```python
from build123d import *

# Parameters (mm, degrees)
ESQUISSE1_R             = 4
BASE_EXTRUSION_DEPTH    = 25
ESQUISSE2_R             = 6.5
BOSS_EXTRU_1_DEPTH      = 8
ENL_V_MAT_EXTRU_1_DEPTH = 3.5
CONG_2_R                = 0.5
CHANFREIN1_SIZE         = 0.5


with BuildPart() as part:
    # Esquisse1 → Base-Extrusion (new body)
    with BuildSketch(Plane.XY):
        Circle(ESQUISSE1_R)
    extrude(amount=BASE_EXTRUSION_DEPTH)

    # Esquisse2 → Boss.-Extru.1 (add)
    with BuildSketch(Plane.XY.offset(25)):
        Circle(ESQUISSE2_R)
    extrude(amount=BOSS_EXTRU_1_DEPTH)

    # Esquisse3 → Enlèv. mat.-Extru.1 (cut)
    with BuildSketch(Plane.XY.offset(33)):
        Polygon((-1.732050808, 3), (1.732050808, 3), (3.464101615, 0), (1.732050808, -3), (-1.732050808, -3), (-3.464101615, 0), align=None)
    extrude(amount=-ENL_V_MAT_EXTRU_1_DEPTH, mode=Mode.SUBTRACT)

    # Congé2
    cong_2_edges = [part.edges().sort_by_distance(p)[0] for p in [
        (-6.5, 0, 33),
    ]]
    fillet(cong_2_edges, radius=CONG_2_R)

    # Chanfrein1
    chanfrein1_edges = [part.edges().sort_by_distance(p)[0] for p in [
        (-4, 0, 0),
    ]]
    chamfer(chanfrein1_edges, length=CHANFREIN1_SIZE)


solid = part.part
```
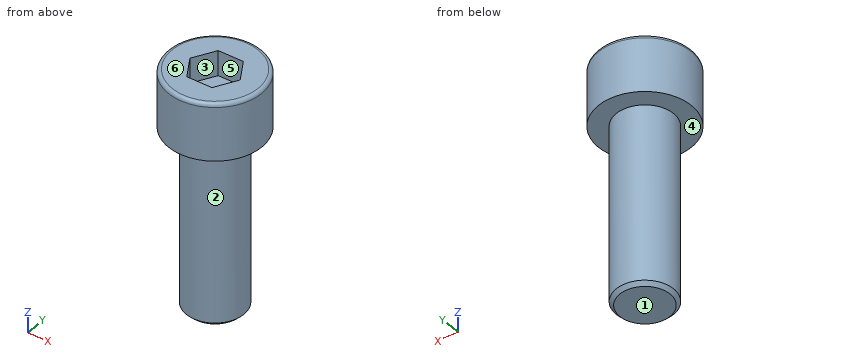
The listing builds one solid part. Answer for the finished solid, in the listing's coordinates (mm). Face numbers are marked on the shaded views. A direction names the side the tool comes from. Give positions to 0.01 mm unless a question says otherwise; leave off trailing zeros. Order: outer loops, then holes, each group sorted by start corner. A loop starts at its lowest first (then second) coordinate and runs counter-clockwise, first axis right, second up.
Item 1: Given pin 1 Ø1.8 at (x, y) = (-0.5, -1) entering from +Z; pin 2 Ø1 at (x, z) = (0.5, 19.5) entering from -Y, each flat-ended and moving along its own axis, determine where each tip first touches the part or whether it passes through.
From the geometry:
pin 1: stops at z = 29.5
pin 2: stops at y = -4
Item 2: The part is cut by section B-B, the plane z = 16. Give the vertices of the cut face in (x, y).
From the geometry:
outline: circle Ø8 at (0, 0)
Item 3: Find the intervals of material crossed by probe 1 along Z at (x, y) = (0.5, -4); probe 2 along Z at (x, y) = (-1, -2); probe 3 along X at (y, z) = (2, 10), in increasing order.
From the geometry:
probe 1: z = 25 to 33
probe 2: z = 0 to 29.5
probe 3: x = -3.46 to 3.46
Item 4: For a pull along X with two mould halves and no side action, classify the marked faces 1, 2 and 3 as pulls with the +X half, pulls with the -X half, needs draft (parallel to the pull), parting line crosses it, or undercut.
From the geometry:
face 1: needs draft
face 2: parting line crosses it
face 3: undercut
Item 5: The part is cut by section A-A, the plane x = 0. Give the vertices of the cut face in (y, z), and give its area (3 significant figures).
From the geometry:
outline: (-6.5, 25) - (-4, 25) - (-4, 0.5) - (-3.5, 0) - (3.5, 0) - (4, 0.5) - (4, 25) - (6.5, 25) - (6.5, 32.5) arc R0.5 ccw to (6, 33) - (3, 33) - (3, 29.5) - (-3, 29.5) - (-3, 33) - (-6, 33) arc R0.5 ccw to (-6.5, 32.5) - close
area: 283 mm2
Item 6: Which of the six approach directions +Z, -Z, +X, -X, +Y, -Y give full straight-line access (tool end or side, diameter ignored) to the marked faces 4, 5 and 6?
From the geometry:
face 4: -Z
face 5: +Z
face 6: +Z, +X, -X, +Y, -Y
